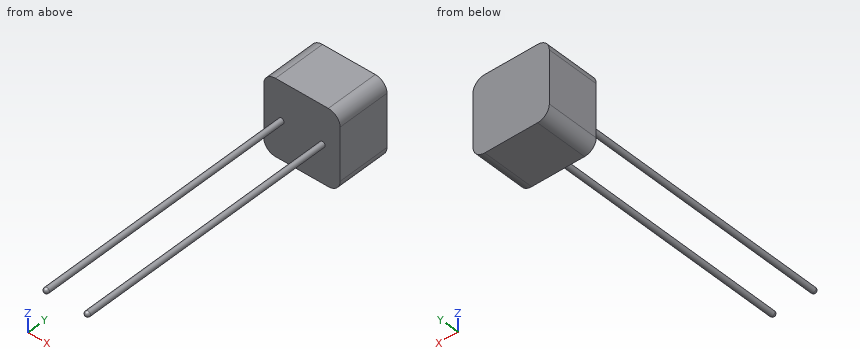
Autodesk Inventor part; units mm, degrees
ref_plane "YZ Plane" through (0, 0, 0) normal (1, 0, 0) x (0, 1, 0)
ref_plane "XZ Plane" through (0, 0, 0) normal (0, 1, 0) x (-1, 0, 0)
ref_plane "XY Plane" through (0, 0, 0) normal (0, 0, 1) x (1, 0, 0)
sketch "Sketch1" plane through (0, 0, 0) normal (0, 1, 0) x (-1, 0, 0)
  line L0 (2.25, 3.25) -> (-2.25, 3.25)
  line L1 (-3.25, 2.25) -> (-3.25, -2.25)
  line L2 (-2.25, -3.25) -> (2.25, -3.25)
  line L3 (3.25, -2.25) -> (3.25, 2.25)
  line L4 (3.25, 3.25) -> (-3.25, -3.25) construction
  line L5 (-3.25, 3.25) -> (3.25, -3.25) construction
  arc A0 (-3.25, -2.25) -> (-2.25, -3.25) centre (-2.25, -2.25) ccw
  arc A1 (2.25, -3.25) -> (3.25, -2.25) centre (2.25, -2.25) ccw
  arc A2 (3.25, 2.25) -> (2.25, 3.25) centre (2.25, 2.25) ccw
  arc A3 (-2.25, 3.25) -> (-3.25, 2.25) centre (-2.25, 2.25) ccw
  point P0 (0, 0)
  dimension "d0" = 6.5
  dimension "d1" = 6.5
  dimension "d4" = 1
extrude "Extrusion1" add sketch "Sketch1" along normal mid plane 4.5
sketch "Sketch4" plane through (0, 0, 0) normal (0, 0, 1) x (1, 0, 0)
  line L0 (-1.75, -25) -> (-1.75, -2.25)
  line L1 (-1.75, -2.25) -> (-1.5182, -2.25)
  line L2 (-1.5182, -2.25) -> (-1.5182, -24.7516)
  arc A0 (-1.75, -25) -> (-1.5182, -24.7516) centre (-1.7559, -24.7621) ccw
  point P0 (0, 0)
revolve "Revolution1" add sketch "Sketch4" angle 360 about axis through (-1.75, -25, 0) along (0, 1, 0)
pattern_linear "Rectangular Pattern3" count 2 spacing 3.5 along (1, 0, 0) of "Revolution1"
properties part number "A54"
Read the model definition and answer for the solid it produces. Units are mm, in the model's axes. Round coordinates to 2 decimals unless told otherwise and drop trailing zeros. Order: outer loops, then holes, each group sorted by start corner. A loop starts at its lowest first (then second) coordinate and runs counter-clockwise, first axis right, second up.
1) The part is cut by section A-A on y = 0. Write down the section's boundary in (x, z), plus the area to 3 significant figures.
2) The part is cut by section D-D on x = 0.75. Write down the section's boundary in (y, z), plus the area to 4 significant figures.
3) The part is cut by section C-C on z = 0.75. Write down the section's boundary in (x, y).
4) Straight lines are drawn through the part: L1, parallel to X at y = -4, z = 0; L2, parallel to Z at x = 1.75, y = -2.5; L3, parallel to Y at x = 2, z = -0.75. For each, find the intervals that lie inside material, in ascending order.
5) The part is cut by section B-B on y = -18. Write down the section's boundary in (x, z).
6) Flat-ended cylindrical pins translate along their axes: pin 1 (1.5 mm diameter, centred on y = -9.5, z = 0, fed in from -X); pin 2 (1 mm diameter, centred on x = -0.5, z = 1.5, fed in from -Y); pin 3 (1.5 mm diameter, centred on x = 1, y = -18.5, fed in from +Z); pin 4 (1.5 mm diameter, centred on x = -0.5, y = -9, fed in from +Z). Find the tip coordinate at first contact, or state that the pin passes through.
Resolved:
1. outline: (-3.25, -2.25) arc R1 ccw to (-2.25, -3.25) - (2.25, -3.25) arc R1 ccw to (3.25, -2.25) - (3.25, 2.25) arc R1 ccw to (2.25, 3.25) - (-2.25, 3.25) arc R1 ccw to (-3.25, 2.25) - close
1. area: 41.4 mm2
2. outline: (-2.25, -3.25) - (2.25, -3.25) - (2.25, 3.25) - (-2.25, 3.25) - close
2. area: 29.25 mm2
3. outline: (-3.25, -2.25) - (3.25, -2.25) - (3.25, 2.25) - (-3.25, 2.25) - close
4. L1: x = -1.98 to -1.52, 1.52 to 1.98
4. L2: z = -0.23 to 0.23
4. L3: y = -2.25 to 2.25
5. outline: circle Ø0.46 at (-1.75, 0); circle Ø0.46 at (1.75, 0)
6. pin 1: stops at x = -1.98
6. pin 2: stops at y = -2.25
6. pin 3: stops at z = 0.23
6. pin 4: passes through
